Autodesk Inventor part; units mm, degrees
ref_plane "工作平面1" through (3, 0, 0) normal (1, 0, 0) x (0, 0, -1)
ref_plane "工作平面3" through (-79.3581, 2.5, -42.5) normal (0, 0, 1) x (1, 0, 0)
ref_plane "工作平面5" through (3, 0, 0) normal (-1, 0, 0) x (0, 0, 1)
sketch "草圖1" plane through (0, 0, 0) normal (1, 0, 0) x (0, 1, 0)
  line L0 (0, 0) -> (5, 0)
  line L1 (5, 0) -> (5, -85)
  line L2 (5, -85) -> (0, -85)
  line L3 (0, -85) -> (0, 0)
  dimension "d0" = 5
  dimension "d1" = 85
extrude "擠出1" add sketch "草圖1" along normal blind 6
fillet "圓角1" radius 2.5 2 edges at (3, 5, 0) (3, 0, 0)
hole "孔1" at (6, 2.5, -2.5) direction (-1, 0, 0) diameter 3 end through all
fillet "圓角2" radius 2.5 2 edges at (3, 5, -85) (3, 0, -85)
hole "孔2" at (6, 2.5, -82.5) direction (-1, 0, 0) diameter 3 end through all
sketch "草圖2" plane through (6, 0, 0) normal (1, 0, 0) x (0, 0, -1)
  line L0 (0, -1) -> (0, 6)
  line L1 (0, -1) -> (0, 6)
  line L2 (120, 0) -> (-20, 0)
  circle A0 centre (82.5, 2.5) radius 1.5
  circle A1 centre (2.5, 2.5) radius 1.5
  arc A2 (82.5, 0) -> (82.5, 5) centre (82.5, 2.5) ccw
  line L3 (82.5, 5) -> (2.5, 5)
  arc A3 (2.5, 5) -> (2.5, 0) centre (2.5, 2.5) ccw
  line L4 (2.5, 0) -> (82.5, 0)
  circle A4 centre (98.5, 2.5) radius 1.5
  circle A5 centre (82.5, 2.5) radius 1.5
  line L5 (84.5, 4) -> (98.5, 4)
  line L6 (98.5, 4) -> (98.5, 1)
  line L7 (98.5, 1) -> (84.5, 1)
  point P0 (0, 0)
  dimension "d24" = 3
  dimension "d25" = 16
extrude "擠出2" add sketch "草圖2" against normal blind 5 contours A2 L5 A4 L7 | L6 A4 | A4 L6
ref_plane "工作平面1" through (3, 0, 0) normal (1, 0, 0) x (0, 0, -1)
sketch "草圖3" plane through (3, 0, 0) normal (1, 0, 0) x (0, 0, -1)
  arc A0 (98.5, 1) -> (98.5, 4) centre (98.5, 2.5) ccw
  line L0 (98.5, 1) -> (102.8586, 1)
  line L1 (102.8586, 1) -> (102.8586, 5.3685)
  line L2 (102.8586, 5.3685) -> (98.5, 5.3685)
  line L3 (98.5, 5.3685) -> (98.5, 1)
  point P0 (0, 0)
extrude "擠出3" cut sketch "草圖3" along normal mid plane 6
sketch "草圖4" plane through (3, 0, 0) normal (1, 0, 0) x (0, 0, -1)
  line L0 (98.5, 4) -> (98.5, 1)
  arc A0 (98.5, 0) -> (98.5, 5) centre (98.5, 2.5) ccw
  line L1 (98.5, 5) -> (98.5, 0)
  point P0 (0, 0)
  dimension "d30" = 5
revolve "迴轉1" add sketch "草圖4" angle 360 about axis through (3, 5, -98.5) along (0, -1, 0)
ref_plane "工作平面3" through (-79.3581, 2.5, -42.5) normal (0, 0, 1) x (1, 0, 0)
ref_plane "工作平面2" through (-79.3581, 2.5, -2.5) normal (0, 0, 1) x (1, 0, 0)
mirror "鏡射1" about plane through (-79.3581, 2.5, -42.5) normal (0, 0, 1) of "迴轉1", "擠出2", "擠出3"
sketch "草圖5" plane through (0, 0, 0) normal (-1, 0, 0) x (0, 0, 1)
  circle A0 centre (-82.5, 2.5) radius 1.5
  arc A1 (-82.5, 5) -> (-82.5, 0) centre (-82.5, 2.5) ccw
  line L0 (-82.5, 0) -> (-2.5, 0)
  arc A2 (-2.5, 0) -> (-2.5, 5) centre (-2.5, 2.5) ccw
  line L1 (-2.5, 5) -> (-82.5, 5)
  circle A3 centre (-2.5, 2.5) radius 1.5
  line L2 (-82.5, 0) -> (-111.7443, 0)
  line L3 (-111.7443, 0) -> (-111.7443, 9.7981)
  line L4 (-111.7443, 9.7981) -> (-82.5, 9.7981)
  line L5 (-82.5, 9.7981) -> (-82.5, 5)
  point P0 (0, 0)
extrude "擠出4" cut sketch "草圖5" against normal blind 68 contours A1 L2 L3 L4 L5
sketch "草圖6" plane through (6, 0, 0) normal (1, 0, 0) x (0, 0, -1)
  line L0 (-100.5, 5.0204) -> (-0.5, 5.0204)
  line L1 (-0.5, 5.0204) -> (-0.5, -3.8226)
  line L2 (-0.5, -3.8226) -> (-100.5, -3.8226)
  line L3 (-100.5, -3.8226) -> (-100.5, 5.0204)
  circle A0 centre (2.5, 2.5) radius 1.5
  point P0 (0, 0)
  dimension "d36" = 100
  dimension "d37" = 3
extrude "擠出5" cut sketch "草圖6" against normal blind 30.5 contours L0 L1 L2 L3
sketch "草圖7" plane through (6, 0, 0) normal (1, 0, 0) x (0, 0, -1)
  line L0 (-0.5, 4) -> (-0.5, 1)
  line L1 (-0.5, 4) -> (-9, 4)
  line L2 (-9, 4) -> (-9, 1)
  line L3 (-9, 1) -> (-0.5, 1)
  line L4 (-0.5, 1) -> (-0.5, 4)
  point P0 (0, 0)
  dimension "d40" = 8.5
extrude "擠出6" add sketch "草圖7" against normal up to surface (5 mm away)
ref_plane "工作平面5" through (3, 0, 0) normal (-1, 0, 0) x (0, 0, 1)
sketch "草圖8" plane through (3, 0, 0) normal (-1, 0, 0) x (0, 0, 1)
  line L0 (9, 4) -> (9, 1)
  arc A0 (9, 0) -> (9, 5) centre (9, 2.5) ccw
  line L1 (9, 5) -> (9, 0)
  point P0 (0, 0)
  dimension "d43" = 5
revolve "迴轉2" add sketch "草圖8" angle 360 about axis through (3, 5, 9) along (0, -1, 0)
ref_plane "工作平面4" through (3, 0, -85) normal (-1, 0, 0) x (0, 0, 1)
properties part number "支架3"
Build history of the part. All positions in model axes, mm. Round coordinates to 2 decimals unless told otherwise and drop trailing zeros. Order: outer loops, then holes, each group sorted by start corner. A loop starts at its lowest first (then second) coordinate and runs counter-clockwise, first axis right, second up. Notation, with made-up numbers: (24.25, -34.5) -> (34.25, -34.5) arc R21 ccw to (34.25, -12.5) -> close; hole circle Ø11 at (87.25, 74.5). An arc over 180 degrees is marked (long way). Answer in a Markdown table with one row per item.
1) Band-saw the part on A-A on x = 3.95. Give the cut face in (y, z), and give its area (3 significant figures).
Values:
| item | result |
|---|---|
| outline | (0, -82.5) arc R2.5 ccw to (5, -82.5) -> (5, -2.5) arc R2.5 ccw to (4, -0.5) -> (4, 7.24) arc R2.31 ccw (long way) to (1, 7.24) -> (1, -0.5) arc R2.5 ccw to (0, -2.5) -> close; hole circle Ø3 at (2.5, -82.5); hole circle Ø3 at (2.5, -2.5) |
| area | 443 mm2 |
2) Wall check: L1, parallel to Z at x = 3.3, y = 2.5; L2, parallel to Y at x = 4.55, z = -82.5; L3, parallel to Z at x = 2, y = 2.5. Give the ranges that are in metal, low to high.
Values:
| item | result |
|---|---|
| L1 | -85 to -84, -81 to -4, -1 to 11.48 |
| L2 | 0 to 1, 4 to 5 |
| L3 | -85 to -84, -81 to -4, -1 to 11.29 |
3) Band-saw the part on B-B on z = 3.5. Give the cut face in (x, y), and give its area (3 significant figures).
Values:
| item | result |
|---|---|
| outline | (1, 1) -> (6, 1) -> (6, 4) -> (1, 4) -> close |
| area | 15.0 mm2 |
4) Mould opens along Z. For faces 1 (the cylindrical face through (3, 2.6, -85)), 2 (the cylindrical face through (2.96, 2.05, -83.93)), 3 (the flat face through (0, 2, -42)) say: released by +Z, released by -Z, zero draft, split by the parting line, or undercut.
Values:
| item | result |
|---|---|
| face 1 | released by -Z |
| face 2 | undercut |
| face 3 | zero draft |
5) Pin check, flat tips, straight feed: P1, Ø0.8, axis at x = 5.5, y = 2.5, coming from the +Z side; P2, Ø1.5, axis at x = 3, z = 2.5, coming from the +Y side. Stop position of each tip, or through.
Values:
| item | result |
|---|---|
| P1 | z = 10.36 |
| P2 | y = 4 |
